Check sheet for the modelled part. Datum: model origin and axes. Units: mm. Face numbers are marked on the shaded views. A direction names the side the tool comes from. Round coordinates to 2 decimals unless told otherwise and drop trailing zeros. Write each loop counter-clockwise with the first axis right and the second up, starting at its lowest first coordinate (ties: lowest second). Pieces come first, ordered by that corner, then holes.
Item 1: Material ranges on line 1 along Y through (x, z) = (-58, 1.2); line 2 along Y through (x, z) = (15, 35); line 3 along X through (y, z) = (-15.5, 1.3), recorded low to high.
Item 2: Section check B-B, the plane x = -42.5. Record the cut outline in (y, z), plus the area to 3 significant figures.
Item 3: Section check D-D, the plane y = 15.5. Record the cut outline in (x, z), plus the area to 3 significant figures.
Item 4: Set-up check for the marked faces 1, 2, 3, 4 and 5: record each of +Z, -Z, +X, -X, +Y, -Y from which the full face is reachable in a straight line by a thin tool's end or side.
Item 5: Section check C-C, the plane y = 0. Record the cut outline in (x, z), plus the area to 3 significant figures.
Item 6: Depth check by flat-ended pin: pin 1 (24.5 mm diameter, centred on x = 45, z = 83, fed in from -Y); pin 2 (3 mm diameter, centred on y = 17.5, z = 68.5, fed in from -X); pin 3 (12 mm diameter, centred on y = 17.5, z = 82, fed in from +X). Enter the tip coordinate at first touch or a pass-through.
Item 7: Release check for a two-part mould opening along Y. For the marked faces 6, 7 and 8 record: pulls with the +Y half, pulls with the -Y half, needs draft (parallel to the pull), parting line crosses it, or undercut.
Item 8: Section check A-A, the plane z = 17. Record the cut outline in (x, y), plus the area to 3 significant figures.
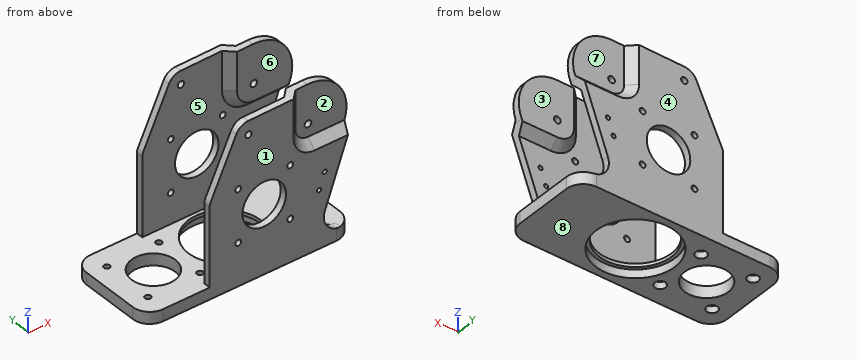
from build123d import *

# Parameters (mm, degrees)
SKETCH_2_R                 = 23.499999999999854
SKETCH_2_R_2               = 12.9999999999999
SKETCH_2_R_3               = 1.7499999999999183
EXTRUDE_1_DEPTH            = 7
SKETCH_5_R                 = 1.2499999999997513
SKETCH_5_R_2               = 1.9999999999997797
SKETCH_5_R_3               = 12.9999999999999
SKETCH_5_R_4               = 1.7500000000003624
SKETCH_5_R_5               = 1.9000000000000128
EXTRUDE_3_DEPTH            = 4
EXTRUDE_START              = -2
SKETCH_6_R                 = 23.499999999999854
SKETCH_6_R_2               = 21.49999999999985
EXTRUDE_4_DEPTH            = 2
FILLET_1_R                 = 10
SKETCH_7_R                 = 3.2500000000000013
SKETCH_7_R_2               = 3.2500000000000004
SKETCH_7_R_3               = 3.250000000000001
CUT_EXTRUDE_4_DEPTH        = 4
SKETCH_18_R                = 1.999999999999777
EXTRUDE_7_DEPTH            = 5
CUT_EXTRUDE_5_DEPTH        = 5
CHAMFER_8_SIZE             = 5
CHAMFER_8_OF_MIRROR_2_SIZE = 5


with BuildPart() as part:
    # 草图2 → 凸台-拉伸1 (new body)
    with BuildSketch(Plane.XY):
        Polygon((-68.50000000000378, -27.499999999999968), (54.94017961354203, -27.499999999999968), (54.94017961354159, 27.4999999999998), (-68.5000000000029, 27.499999999999968), align=None)
        Circle(SKETCH_2_R, mode=Mode.SUBTRACT)
        with Locations((-42.50000000000354, -1.22125e-12)):
            Circle(SKETCH_2_R_2, mode=Mode.SUBTRACT)
        with Locations((-27.000000000003688, 15.499999999998737)):
            Circle(SKETCH_2_R_3, mode=Mode.SUBTRACT)
        with Locations((-27.000000000005464, -15.500000000002178)):
            Circle(SKETCH_2_R_3, mode=Mode.SUBTRACT)
        with Locations((-58.00000000000427, -15.500000000002068)):
            Circle(SKETCH_2_R_3, mode=Mode.SUBTRACT)
        with Locations((-58.00000000000294, 15.499999999998737)):
            Circle(SKETCH_2_R_3, mode=Mode.SUBTRACT)
    extrude(amount=EXTRUDE_1_DEPTH)

    # 草图5 → 凸台-拉伸3 (add)
    with BuildSketch(Plane(origin=(3.71e-14, 27.499999999999876, 0), x_dir=(1, -1.35e-15, 0), z_dir=(1.35e-15, 1, 0))):
        with BuildLine():
            Line((-30.57625495627559, -6.9999999999999964), (47.52563316823275, -6.999999999999941))
            ThreePointArc((47.52563316823275, -6.999999999999941), (39.334112738152676, -11.264235618194132), (38.128706945095715, -20.420201391282454))
            Line((38.128706945095715, -20.420201391282454), (53.20718018719004, -61.84796671962179))
            ThreePointArc((53.20718018719004, -61.84796671962179), (51.05071212212322, -83.63735224169075), (31.628764590502435, -93.74752682099374))
            Line((31.628764590502435, -93.74752682099374), (-7.596215432832855, -93.11432687715183))
            ThreePointArc((-7.596215432832855, -93.11432687715183), (-11.801401356788567, -91.83948575225449), (-14.698924987474284, -88.53597771406503))
            Line((-14.698924987474284, -88.53597771406503), (-30.096151777816445, -55.98323269965879))
            ThreePointArc((-30.096151777816445, -55.98323269965879), (-30.454752886360815, -54.940915116534505), (-30.576254956274703, -53.84535227208149))
            Line((-30.576254956274703, -53.84535227208149), (-30.57625495627559, -6.9999999999999964))
        make_face()
        with Locations(Location((34.72674141312202, -34.00000000000005, 0), (0, 0, 90))):
            Circle(SKETCH_5_R, mode=Mode.SUBTRACT)
        with Locations(Location((38.04433676266059, -43.11501843644486, 0), (0, 0, 90))):
            Circle(SKETCH_5_R, mode=Mode.SUBTRACT)
        with Locations(Location((32.00000000000001, -70.75052301026328, 0), (0, 0, 90))):
            Circle(SKETCH_5_R_2, mode=Mode.SUBTRACT)
        with Locations(Location((1.9479617995710048, -40.698484809835, 0), (0, 0, 90))):
            Circle(SKETCH_5_R_3, mode=Mode.SUBTRACT)
        with Locations(Location((-13.552038200428397, -56.19848480983506, 0), (0, 0, 90))):
            Circle(SKETCH_5_R_4, mode=Mode.SUBTRACT)
        with Locations(Location((17.447961799570404, -56.198484809835, 0), (0, 0, 90))):
            Circle(SKETCH_5_R_4, mode=Mode.SUBTRACT)
        with Locations(Location((17.447961799569516, -25.198484809834156, 0), (0, 0, 90))):
            Circle(SKETCH_5_R_4, mode=Mode.SUBTRACT)
        with Locations(Location((-13.552038200430173, -25.19848480983421, 0), (0, 0, 90))):
            Circle(SKETCH_5_R_4, mode=Mode.SUBTRACT)
        with Locations(Location((-7.467090073007844, -85.11536902994133, 0), (0, 0, 90))):
            Circle(SKETCH_5_R_5, mode=Mode.SUBTRACT)
    extrude_3 = extrude(amount=-EXTRUDE_3_DEPTH)

    # 草图6 → 凸台-拉伸4 (add)
    with BuildSketch(Plane.XY.offset(7).offset(EXTRUDE_START)):
        Circle(SKETCH_6_R)
        Circle(SKETCH_6_R_2, mode=Mode.SUBTRACT)
    extrude(amount=EXTRUDE_4_DEPTH)

    # 镜向1: 凸台-拉伸3 across plane
    add(extrude_3.mirror(Plane.ZX))

    # 圆角1
    fillet_1_edges = [part.edges().sort_by_distance(p)[0] for p in [
        (-68.5000000000029, 27.499999999999968, 3.5),
        (54.94017961354159, 27.4999999999998, 3.5),
        (54.94017961354203, -27.499999999999968, 3.5),
        (-68.50000000000378, -27.499999999999968, 3.5),
    ]]
    fillet(fillet_1_edges, radius=FILLET_1_R)

    # 草图7 → 切除-拉伸4 (cut)
    with BuildSketch(Plane.XY):
        with Locations((-58.00000000000294, 15.499999999998737)):
            Circle(SKETCH_7_R)
        with Locations((-27.000000000003688, 15.499999999998737)):
            Circle(SKETCH_7_R_2)
        with Locations((-27.000000000005464, -15.500000000002178)):
            Circle(SKETCH_7_R_2)
        with Locations((-58.00000000000427, -15.500000000002068)):
            Circle(SKETCH_7_R_3)
    extrude(amount=CUT_EXTRUDE_4_DEPTH, mode=Mode.SUBTRACT)

    # 草图18 → 凸台-拉伸7 (add)
    with BuildSketch(Plane(origin=(3.17e-14, -23.499999999999826, -1.641e-13), x_dir=(1, 1.35e-15, 0), z_dir=(-1.35e-15, 1, 6.98e-15))):
        with BuildLine():
            Line((32.00000000000008, -55.750523010263095), (50.98789220271744, -55.750523010263095))
            Line((50.98789220271744, -55.750523010263095), (53.20718018719011, -61.847966719621596))
            ThreePointArc((53.20718018719011, -61.847966719621596), (51.05071212212356, -83.63735224169073), (31.62876459050252, -93.74752682099322))
            Line((31.62876459050252, -93.74752682099322), (17.000000000000078, -93.51137799665558))
            Line((17.000000000000078, -93.51137799665558), (17.000000000000078, -70.7505230102631))
            ThreePointArc((17.000000000000078, -70.7505230102631), (21.393398282201865, -60.14392129246488), (32.00000000000008, -55.750523010263095))
        make_face()
        with Locations(Location((32.00000000000008, -70.7505230102631, 0), (0, 0, 90))):
            Circle(SKETCH_18_R, mode=Mode.SUBTRACT)
    extrude_7 = extrude(amount=EXTRUDE_7_DEPTH)

    # 草图9 → 切除-拉伸5 (cut)
    with BuildSketch(Plane.XZ.offset(27.499999999999968)):
        with BuildLine():
            Line((19.50000000000005, 70.75052301026328), (19.500000000000046, 93.55173492886229))
            Line((19.500000000000046, 93.55173492886229), (31.628764590502485, 93.74752682099341))
            ThreePointArc((31.628764590502485, 93.74752682099341), (51.05071212212326, 83.63735224169075), (53.207180187190076, 61.84796671962179))
            Line((53.207180187190076, 61.84796671962179), (51.89781777573519, 58.25052301026329))
            Line((51.89781777573519, 58.25052301026329), (32.00000000000004, 58.25052301026329))
            ThreePointArc((32.00000000000004, 58.25052301026329), (23.161165235168202, 61.91168824543144), (19.50000000000005, 70.75052301026328))
        make_face()
    cut_extrude_5 = extrude(amount=-CUT_EXTRUDE_5_DEPTH, mode=Mode.SUBTRACT)

    # 倒角8
    chamfer_8_edges = [part.edges().sort_by_distance(p)[0] for p in [
        (41.94890888786762, -22.499999999999968, 58.25052301026329),
        (23.161165235168205, -22.499999999999968, 61.91168824543144),
        (19.50000000000005, -22.499999999999968, 82.15112896956279),
        (41.49394610135879, -18.50000000000016, 55.75052301026297),
        (21.39339828220189, -18.500000000000217, 60.14392129246475),
        (17.000000000000103, -18.500000000000377, 82.1309505034592),
    ]]
    chamfer(chamfer_8_edges, length=CHAMFER_8_SIZE - 0.0001)  # a hair under: the kernel refuses the full size

    # 镜向2: 凸台-拉伸7, 切除-拉伸5 across plane
    add(extrude_7.mirror(Plane.ZX))
    add(cut_extrude_5.mirror(Plane.ZX), mode=Mode.SUBTRACT)

    # 倒角8 of 镜向2
    chamfer_8_of_mirror_2_edges = [part.edges().sort_by_distance(p)[0] for p in [
        (41.94890888786762, 22.499999999999968, 58.25052301026329),
        (23.161165235168205, 22.499999999999968, 61.91168824543144),
        (19.50000000000005, 22.499999999999968, 82.15112896956279),
        (41.49394610135879, 18.500000000000153, 55.75052301026297),
        (21.39339828220189, 18.500000000000217, 60.14392129246475),
        (17.000000000000103, 18.50000000000038, 82.1309505034592),
    ]]
    chamfer(chamfer_8_of_mirror_2_edges, length=CHAMFER_8_OF_MIRROR_2_SIZE - 0.0001)  # a hair under: the kernel refuses the full size


solid = part.part
Values found:
1. line 1: y = -27.5 to -18.75, -12.25 to 12.25, 18.75 to 27.5
1. line 2: y = -27.5 to -23.5, 23.5 to 27.5
1. line 3: x = -68.5 to -61.25, -54.75 to -30.25, -23.75 to -17.66, 17.66 to 54.94
2. outline: (-27.5, 0) - (-13, 0) - (-13, 7) - (-27.5, 7) - close; (13, 0) - (27.5, 0) - (27.5, 7) - (13, 7) - close
2. area: 203 mm2
3. outline: (-68.5, 0) - (-61.25, 0) - (-61.25, 4) - (-59.75, 4) - (-59.75, 7) - (-68.5, 7) - close; (-56.25, 4) - (-54.75, 4) - (-54.75, 0) - (-30.25, 0) - (-30.25, 4) - (-28.75, 4) - (-28.75, 7) - (-56.25, 7) - close; (-25.25, 4) - (-23.75, 4) - (-23.75, 0) - (-17.66, 0) - (-17.66, 5) - (-14.9, 5) - (-14.9, 7) - (-25.25, 7) - close; (14.9, 5) - (17.66, 5) - (17.66, 0) - (54.94, 0) - (54.94, 7) - (14.9, 7) - close
3. area: 555 mm2
4. face 1: +Z, -Z, +X, -X, -Y
4. face 2: +Z, +X, -Y
4. face 3: +Z, +X, -X
4. face 4: +Z, -Z, +X, -X, +Y
4. face 5: -X
5. outline: (-68.5, 0) - (-55.5, 0) - (-55.5, 7) - (-68.5, 7) - close; (-29.5, 0) - (-23.5, 0) - (-23.5, 5) - (-21.5, 5) - (-21.5, 7) - (-29.5, 7) - close; (21.5, 5) - (23.5, 5) - (23.5, 0) - (54.94, 0) - (54.94, 7) - (21.5, 7) - close
5. area: 361 mm2
6. pin 1: stops at y = -22.5
6. pin 2: stops at x = 21.71
6. pin 3: stops at x = 54.37
7. face 6: undercut
7. face 7: pulls with the +Y half
7. face 8: needs draft
8. outline: (-30.58, -27.5) - (37.53, -27.5) - (37.53, -23.5) - (-30.58, -23.5) - close; (-30.58, 23.5) - (37.53, 23.5) - (37.53, 27.5) - (-30.58, 27.5) - close
8. area: 545 mm2
